Job drawing, mm, ordinate dimensions from the low corner. One solid piece. A direction names the side the tool comes from. Give positions to 0.01 mm unless a question says otherwise; leave off trailing zeros. Loops run counter-clockwise (first coordinate to the right, second up) from the corner with the lowest first, then second, coordinate; pieces in that order, holes last.
Item 1: Saw through at C-C on z = 1. Give the cut face in (x, y), plus the area to 3 significant figures.
Item 2: Drop flat-ended pins along their axis: P1, Ø1.3, axis at y = 3, z = 11.5, coming from the -X side; P2, Ø1.5, axis at x = 14, y = 3.5, coming from the +Z side; P3, Ø1.6, axis at y = 2.5, z = 12.5, coming from the -X side. Give the stop position or say it passes through.
Item 3: Which spindle directions (+Z, -Z, +X, -X, +Y, -Y) get a long thin tool onto all of the face, cutting with end or side? Do the marked faces 4, 5 and 6. Say none if no direction does.
Item 4: Saw through at A-A on y = 0.3. Give the cut face in (x, z).
Item 5: Mould opens along X. For the marked faces 1, 2 and 3 say: released by +X, released by -X, zero draft, split by the parting line, or undercut.
Item 6: Saw through at B-B on x = 15.75. Give the cut face in (y, z).
Item 7: Probe probe 1 along X at (y, z) = (4.5, 11.75); probe 2 along X at (y, z) = (3.15, 10.5); probe 3 along Z at (x, y) = (25.75, 3.9). List the from-to ranges inside material, lowest first.
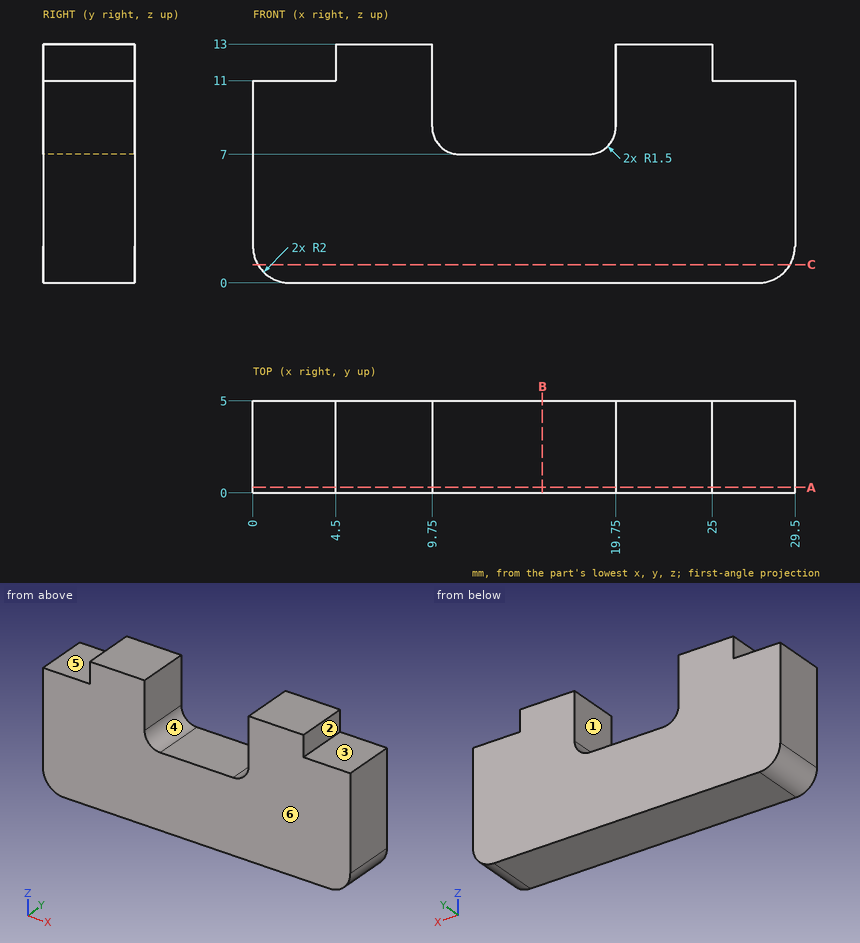
Results below:
1. outline: (0.27, 0) - (29.23, 0) - (29.23, 5) - (0.27, 5) - close
1. area: 145 mm2
2. P1: stops at x = 0
2. P2: stops at z = 7
2. P3: stops at x = 4.5
3. face 4: +Z, +Y, -Y
3. face 5: +Z, -X, +Y, -Y
3. face 6: +Z, -Z, +X, -X, -Y
4. outline: (0, 2) arc R2 ccw to (2, 0) - (27.5, 0) arc R2 ccw to (29.5, 2) - (29.5, 11) - (25, 11) - (25, 13) - (19.75, 13) - (19.75, 8.5) arc R1.5 cw to (18.25, 7) - (11.25, 7) arc R1.5 cw to (9.75, 8.5) - (9.75, 13) - (4.5, 13) - (4.5, 11) - (0, 11) - close
5. face 1: undercut
5. face 2: released by +X
5. face 3: zero draft
6. outline: (0, 0) - (5, 0) - (5, 7) - (0, 7) - close
7. probe 1: x = 4.5 to 9.75, 19.75 to 25
7. probe 2: x = 0 to 9.75, 19.75 to 29.5
7. probe 3: z = 0 to 11
